Autodesk Inventor part; units mm, degrees
ref_plane "YZ Plane" through (0, 0, 0) normal (1, 0, 0) x (0, 1, 0)
ref_plane "XZ Plane" through (0, 0, 0) normal (0, 1, 0) x (-1, 0, 0)
ref_plane "XY Plane" through (0, 0, 0) normal (0, 0, 1) x (1, 0, 0)
sketch "Skizze1" plane through (0, 0, 0) normal (0, 0, 1) x (1, 0, 0)
  line L0 (0, 80) -> (24, 80)
  line L1 (24, 80) -> (24, -80)
  line L2 (24, -80) -> (0, -80)
  line L3 (0, -80) -> (0, 80)
  line L4 (24, 40) -> (124, 40)
  line L5 (124, 40) -> (124, -40)
  line L6 (124, -40) -> (24, -40)
  line L7 (24, -40) -> (24, 40)
  point P0 (0, 0)
  point P1 (24, 0)
  point P2 (0, 0)
  point P3 (94, 0)
  point P4 (124, 0)
  dimension "d0" = 160
  dimension "d1" = 24
  dimension "d2" = 124
  dimension "d3" = 80
  dimension "d4" = 94
extrude "Extrusion1" add sketch "Skizze1" along normal mid plane 160 contours L0 L1 L2 L3
sketch "Skizze2" plane through (24, -80, 80) normal (1, 0, 0) x (0, 0, -1)
  line L0 (0, 160) -> (30, 160)
  line L1 (30, 160) -> (30, 130)
  line L2 (30, 130) -> (0, 130)
  line L3 (0, 130) -> (0, 160)
  point P0 (80, 80)
  dimension "d19" = 30
  dimension "d20" = 30
extrude "Extrusion4" cut sketch "Skizze2" against normal blind 9
pattern_circular "Runde Anordnung1" count 4 over 360 about axis through (-10, 0, 0) along (1, 0, 0) of "Extrusion4"
sketch "Skizze3" plane through (24, 50, 50) normal (1, 0, 0) x (0, 0, -1)
  line L0 (-15, 15) -> (115, 15)
  line L1 (115, 15) -> (115, -115)
  line L2 (115, -115) -> (-15, -115)
  line L3 (-15, -115) -> (-15, 15)
  line L4 (-15, 15) -> (115, -115) construction
  line L5 (115, 15) -> (-15, -115) construction
  point P0 (50, -50)
  dimension "d26" = 130
  dimension "d27" = 130
hole "Bohrung2" at (24, 65, 65) at (24, -65, 65) at (24, 65, -65) at (24, -65, -65) direction (-1, 0, 0) diameter 10.5 end through all
fillet "Rundung2" radius 15 4 edges at (7.5, 80, -80) (7.5, -80, -80) (7.5, -80, 80) (7.5, 80, 80)
fillet "Rundung3" radius 10 4 edges at (19.5, -50, 50) (19.5, -50, -50) (19.5, 50, -50) (19.5, 50, 50)
sketch "Skizze4" plane through (24, -50, 80) normal (1, 0, 0) x (0, 0, -1)
  line L0 (130, 130) -> (30, 130)
  line L1 (130, -30) -> (30, -30)
  line L2 (130, 130) -> (30, 130)
  line L3 (30, 130) -> (30, -30)
  line L4 (30, -30) -> (130, -30)
  line L5 (130, -30) -> (130, 130)
  line L6 (130, 110) -> (130, 130)
  line L7 (30, 130) -> (130, 130)
  line L8 (130, 130) -> (130, 120)
  line L9 (130, 120) -> (30, 120)
  line L10 (30, 120) -> (30, 130)
  point P0 (80, 50)
  dimension "d37" = 10
extrude "Extrusion5" add sketch "Skizze4" along normal blind 50 contours L5 L9 L3 L0
sketch "Skizze5" plane through (24, 70, -50) normal (0, -1, 0) x (1, 0, 0)
  circle A0 centre (25, 25) radius 5
  circle A1 centre (25, 75) radius 5
  point P0 (-24, 50)
  dimension "d40" = 10
  dimension "d41" = 10
extrude "Extrusion6" cut sketch "Skizze5" against normal blind 10
chamfer "Fase1" distance 2 angle 45 2 edges at (44, 70, -25) (44, 70, 25)
fillet "Rundung4" radius 1 3 edges at (74, 70, 0) (49, 70, -50) (49, 70, 50)
equation "\"d5\" = d0"
properties part number "Gelenkflansch" material "Stahl AISI 4130"
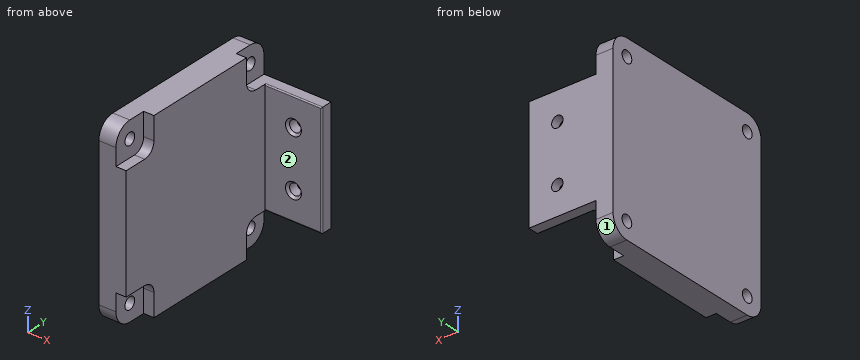
Read the model definition and answer for the solid it produces. Units are mm, in the model's axes. Face numbers are marked on the shaded views. A direction names the side the tool comes from. Round coordinates to 2 decimals unless told otherwise and drop trailing zeros. Order: outer loops, then holes, each group sorted by start corner. A loop starts at its lowest first (then second) coordinate and runs counter-clockwise, first axis right, second up.
1) Flat-ended cylindrical pins translate along their axes: pin 1 (7 mm diameter, centred on x = 19, z = 70.5, fed in from +Y); pin 2 (2.5 mm diameter, centred on x = 21, z = 66, fed in from -Y); pin 3 (10 mm diameter, centred on x = 32.5, y = 74, fed in from +Z). Find the tip coordinate at first contact, or state that the pin passes through.
2) The part is cut by section D-D on x = 28. Write down the section's boundary in (y, z), plus the area to 4 significant figures.
3) For the marked faces 1 and 2, determine the directions among +Z, -Z, +X, -X, +Y, -Y from which every point of the face is accessible in a straight line to the end or side of a thin tool.
4) The part is cut by section B-B on x = 49. Write down the section's boundary in (y, z).
5) The part is cut by section A-A on x = 10. Write down the section's boundary in (y, z), plus the area to 3 significant figures.
6) Straight lines are drawn through the part: L1, parallel to Y at x = 10.75, z = 65; L2, parallel to Z at x = 49, y = 73.5. For each, find the intervals that lie inside material, in ascending order.
7) The part is cut by section C-C on z = 10.5. Write down the section's boundary in (x, y).
Resolved:
1. pin 1: stops at y = 50
1. pin 2: stops at y = -50
1. pin 3: stops at z = 50
2. outline: (70, -49) arc R1 ccw to (71, -50) - (80, -50) - (80, 50) - (71, 50) arc R1 ccw to (70, 49) - close
2. area: 1,000 mm2
3. face 1: -Z, +X, -X, +Y
3. face 2: +Z, -Z, +X, -Y
4. outline: (70, -49) arc R1 ccw to (71, -50) - (80, -50) - (80, -30) - (72, -30) - (70, -32) - close; (70, -18) - (72, -20) - (80, -20) - (80, 20) - (72, 20) - (70, 18) - close; (70, 32) - (72, 30) - (80, 30) - (80, 50) - (71, 50) arc R1 ccw to (70, 49) - close
5. outline: (-80, -65) arc R15 ccw to (-65, -80) - (65, -80) arc R15 ccw to (80, -65) - (80, 65) arc R15 ccw to (65, 80) - (-65, 80) arc R15 ccw to (-80, 65) - close; hole circle Ø10.5 at (-65, -65); hole circle Ø10.5 at (-65, 65); hole circle Ø10.5 at (65, -65); hole circle Ø10.5 at (65, 65)
5. area: 25,100 mm2
6. L1: y = -80 to -70.25, -59.75 to 59.75, 70.25 to 80
6. L2: z = -50 to -30, -20 to 20, 30 to 50
7. outline: (0, -80) - (24, -80) - (24, 70) - (73, 70) arc R1 ccw to (74, 71) - (74, 80) - (0, 80) - close
